Work out the finished part from the listing and answer in its coordinate system (mm). Round coordinates to 2 decimals unless told otherwise and drop trailing zeros. Write each loop counter-clockwise with the first axis right and the second up, starting at its lowest first coordinate (ties: lowest second). Pieces come first, ordered by that corner, then holes. Notation, with made-up numbers: M 12,53.25 L 33,53.25 A21 ccw 33,81.25 Z; hole C 21,-22 d2. An arc over 180 degrees is marked long. Answer in a Markdown table with one row per item.
```python
from build123d import *

# Parameters (mm, degrees)
BOSS_EXTRUDE1_DEPTH = 15.5
BOSS_EXTRUDE2_DEPTH = 11.5
FILLET1_R           = 4


with BuildPart() as part:
    # Sketch3 → Boss-Extrude1 (new body)
    with BuildSketch(Plane(origin=(0, 0, 0), x_dir=(1, 0, 0), z_dir=(0, 1, 0))):
        with BuildLine():
            Line((0, 14.5), (0, 19.5))
            ThreePointArc((0, 19.5), (9.75, 16.887495374), (16.887495374, 9.75))
            Line((16.887495374, 9.75), (12.557368355, 7.25))
            ThreePointArc((12.557368355, 7.25), (7.25, 12.557368355), (0, 14.5))
        make_face()
    extrude(amount=BOSS_EXTRUDE1_DEPTH)

    # Sketch5 → Boss-Extrude2 (add)
    with BuildSketch(Plane.XZ):
        with BuildLine():
            Line((6.078565727, -18.528384676), (16.184371608, -36.032153914))
            ThreePointArc((16.184371608, -36.032153914), (19.75, -34.208003449), (23.112574838, -32.032153914))
            Line((23.112574838, -32.032153914), (13.006768957, -14.528384676))
            ThreePointArc((13.006768957, -14.528384676), (9.75, -16.887495374), (6.078565727, -18.528384676))
        make_face()
    extrude(amount=-BOSS_EXTRUDE2_DEPTH)

    # Fillet1
    # the kernel refuses this fillet: 4 mm, written as the material it takes off along each edge
    with BuildSketch(Plane(origin=(28.112574838, 11.5, -40.692407951), x_dir=(-0.8660254037844415, 0, -0.4999999999999951), z_dir=(-0.49999999999999506, 0, 0.8660254037844415))) as fillet1_piece_1_section:
        with BuildLine():
            CenterArc((FILLET1_R, FILLET1_R), FILLET1_R, 180, 90)
            Line((0, FILLET1_R), (0, 0))
            Line((0, 0), (FILLET1_R, 0))
        make_face()
    fillet1_piece_1 = extrude(amount=40.211611762, mode=Mode.PRIVATE)
    fillet1_piece_1 = fillet1_piece_1 - Plane(origin=(0, 10.592283231, 0), x_dir=(0, 0, -1), z_dir=(0, -1, 0)) * Cylinder(19.5, 97, mode=Mode.PRIVATE)
    add(fillet1_piece_1, mode=Mode.SUBTRACT)
    with BuildSketch(Plane(origin=(1.078565727, 11.5, -9.868130638), x_dir=(0, -1, 0), z_dir=(0.49999999999999506, 0, -0.8660254037844415))) as fillet1_piece_2_section:
        with BuildLine():
            CenterArc((FILLET1_R, -FILLET1_R), FILLET1_R, 90, 90)
            Line((0, -FILLET1_R), (0, 0))
            Line((0, 0), (FILLET1_R, 0))
        make_face()
    fillet1_piece_2 = extrude(amount=40.211611762, mode=Mode.PRIVATE)
    fillet1_piece_2 = fillet1_piece_2 - Plane(origin=(0, 10.592276743, 0), x_dir=(0, 0, -1), z_dir=(0, -1, 0)) * Cylinder(19.5, 97, mode=Mode.PRIVATE)
    add(fillet1_piece_2, mode=Mode.SUBTRACT)


solid = part.part
```
1. The part is cut by section C-C (y = 10.5). Determine the outline of the cut face in (x, z), plus the area to 3 significant figures.
Calculated:
| item | result |
|---|---|
| outline | M 0,-19.5 A19.5 ccw 7.37,-18.05 L 17.41,-35.45 A39.5 ccw 22,-32.81 L 11.95,-15.41 A19.5 ccw 16.89,-9.75 L 12.56,-7.25 A14.5 cw 0,-14.5 Z |
| area | 195 mm² |
2. The part is cut by section D-D (x = 4.75). Determine the outline of the cut face in (y, z), plus the area to 3 significant figures.
Calculated:
| item | result |
|---|---|
| outline | M 0,-18.91 L 15.5,-18.91 L 15.5,-13.7 L 0,-13.7 Z |
| area | 80.8 mm² |
3. Consider line 1 along Z through (x, y) = (1.75, 10.5); line 2 along X through (y, z) = (1, -30.25); line 3 along Z through (x, y) = (12.5, 7.5). Determine where each line is inside the solid, lowest interval first. Write a range as from..to.
Calculated:
| item | result |
|---|---|
| line 1 | z = -19.42..-14.39 |
| line 2 | x = 12.85..22.08 |
| line 3 | z = -29.65..-7.35 |
4. Given pin 1 (5 mm diameter, centred on y = 13, z = -28, fed in from +X); pin 2 (5 mm diameter, centred on x = 18.5, z = -14.5, fed in from -Y); pin 3 (6 mm diameter, centred on x = 17, z = -31.5, fed in from +Y), each flat-ended and moving along its own axis, determine where each tip first touches the part or whether it passes through.
Calculated:
| item | result |
|---|---|
| pin 1 | stops at x = 19.51 |
| pin 2 | passes through |
| pin 3 | stops at y = 11.5 |
5. The part is cut by section A-A (y = 1.5). Determine the outline of the cut face in (x, z), plus the area to 3 significant figures.
Calculated:
| item | result |
|---|---|
| outline | M 0,-19.5 A19.5 ccw 6.08,-18.53 L 16.18,-36.03 A39.5 ccw 23.11,-32.03 L 13.01,-14.53 A19.5 ccw 16.89,-9.75 L 12.56,-7.25 A14.5 cw 0,-14.5 Z |
| area | 250 mm² |
6. Determine the mould class of faces 1 (the cylindrical face through (19.701, 5.67, -34.236)), 2 (the cylindrical face through (7.342, 7.642, -12.504)), 3 (the flat face through (18.13, 3.7, -23.4)) for opening direction Z: released by +Z, released by -Z, zero draft, split by the parting line, or undercut.
Calculated:
| item | result |
|---|---|
| face 1 | released by -Z |
| face 2 | released by +Z |
| face 3 | undercut |
7. The part is cut by section B-B (z = -13.75). Determine the outline of the cut face in (x, y).
Calculated:
| item | result |
|---|---|
| outline | M 4.6,0 L 13.83,0 L 13.83,15.5 L 4.6,15.5 Z |
